Build history of the part. All positions in model axes, mm. Round coordinates to 2 decimals unless told otherwise and drop trailing zeros. Order: outer loops, then holes, each group sorted by start corner. A loop starts at its lowest first (then second) coordinate and runs counter-clockwise, first axis right, second up. Notation, with made-up numbers: (10.25, 9) -> (22.25, 9) arc R11 cw to (22.25, 17) -> close; hole circle Ø2 at (36.25, 58). An arc over 180 degrees is marked (long way). Use a Markdown table: item, result. Add a question column.
Item 1: Slice it at B-B, the plane x = 44.5. Give the cut face in (y, z).
Item 2: Slice it at A-A, the plane x = -4.5. Give the cut face in (y, z).
Item 3: Slice it at C-C, the plane y = -9.5. Give the cut face in (x, z), plus the area to 3 significant figures.
Item 4: Probe L1, parallel to Y at x = 60, z = 0.1; L2, parallel to X at y = -14, z = 0.55; L3, parallel to X at y = -26, z = 0.7. List the from-to ranges inside material, lowest first.
Item 5: Two-plate mould, pull along X, no slides. Class faces 1 (the face through (15.343, -16.242, 0.493)), 2 (the face through (-19.63, 22.23, 0.49)), 3 (the face through (12, -5, 1)): released by +X, released by -X, zero draft, split by the parting line, or undercut.
Item 6: Slice it at D-D, the plane z = 0.65. State how many separate pieces and enclosed holes the cut face has, plus the area to 3 significant figures.
from build123d import *

# Parameters (mm, degrees)
F0_R     = 3.25
F0_W     = 21
F0_H     = 10.2114447155
F0_W_2   = 19.5
F0_H_2   = 5.9798656802
F0_W_3   = 45
F1_DEPTH = 1


# Not quite as in the source:
# - a feature names something its author has since deleted; it is built from what else it names


with BuildPart() as f1:
    # F0 (on Top) → F1 (new body)
    with BuildSketch(Plane.XY):
        Polygon((85.2658590674, -26.4641552444), (85.2658590674, 13.2858447556), (68.2658590674, 13.2858447556), (68.2658590674, -1.2141552444), (68.2658590674, -11.42559996), (68.2658590674, -26.4641552444), (23.2658590674, -26.4641552444), (9.2658590674, -26.4641552444), (9.2658590674, -22.7141552444), (-10.2341409326, -22.7141552444), (-10.2341409326, -26.4641552444), (-24.2341409326, -26.4641552444), (-45.2341409326, -26.4641552444), (-45.2341409326, -11.42559996), (-45.2341409326, -1.2141552444), (-45.2341409326, 13.2858447556), (-59.2341409326, 13.2858447556), (-59.2341409326, -26.4641552444), (-59.2341409326, -36.4641552444), (-24.2341409326, -36.4641552444), (85.2658590674, -36.4641552444), align=None)
        with Locations((-52.2341409326, -19.4641552444)):
            Circle(F0_R, mode=Mode.SUBTRACT)
        with Locations((76.7658590674, -19.4641552444)):
            Circle(F0_R, mode=Mode.SUBTRACT)
        with Locations((-52.2341409326, -0.9641552444)):
            Circle(F0_R, mode=Mode.SUBTRACT)
        with Locations((76.7658590674, -0.9641552444)):
            Circle(F0_R, mode=Mode.SUBTRACT)
        with Locations((-34.7341409326, -6.3198776022)):
            Rectangle(F0_W, F0_H)
        with Locations((-0.4841409326, 5.2757775957)):
            Rectangle(F0_W_2, F0_H_2)
        with Locations((45.7658590674, -6.3198776022)):
            Rectangle(F0_W_3, F0_H)
        Polygon((-24.2341409326, 13.2858447556), (-10.2341409326, 13.2858447556), (-10.2341409326, 26.5358447556), (-59.2341409326, 26.5358447556), (-59.2341409326, 13.2858447556), (-45.2341409326, 13.2858447556), align=None)
        with Locations((-17.2341409326, 20.0358447556)):
            Circle(F0_R, mode=Mode.SUBTRACT)
        Polygon((85.2658590674, 13.2858447556), (85.2658590674, 26.2858447556), (9.2658590674, 26.2858447556), (9.2658590674, 13.2858447556), (23.2658590674, 13.2858447556), (68.2658590674, 13.2858447556), align=None)
        with Locations((15.7658590674, 20.7858447556)):
            Circle(F0_R, mode=Mode.SUBTRACT)
        with Locations((76.7658590674, 20.0358447556)):
            Circle(F0_R, mode=Mode.SUBTRACT)
        Polygon((-10.2341409326, 2.2858447556), (-10.2341409326, 8.2657104358), (-10.2341409326, 13.2858447556), (-24.2341409326, 13.2858447556), (-24.2341409326, -1.2141552444), (-24.2341409326, -11.42559996), (-24.2341409326, -26.4641552444), (-10.2341409326, -26.4641552444), (-10.2341409326, -22.7141552444), align=None)
        with Locations((-17.2341409326, -19.4641552444)):
            Circle(F0_R, mode=Mode.SUBTRACT)
        Polygon((23.2658590674, 13.2858447556), (9.2658590674, 13.2858447556), (9.2658590674, 8.2657104358), (9.2658590674, 2.2858447556), (9.2658590674, -22.7141552444), (9.2658590674, -26.4641552444), (23.2658590674, -26.4641552444), (23.2658590674, -11.42559996), (23.2658590674, -1.2141552444), align=None)
        with Locations((15.7658590674, -19.4641552444)):
            Circle(F0_R, mode=Mode.SUBTRACT)
    extrude(amount=F1_DEPTH)


solid = f1.part
Check sheet entries:
| question | item | result |
|---|---|---|
| 1 | outline | (-36.46, 0) -> (-26.46, 0) -> (-26.46, 1) -> (-36.46, 1) -> close; (-11.43, 0) -> (-1.21, 0) -> (-1.21, 1) -> (-11.43, 1) -> close; (13.29, 0) -> (26.29, 0) -> (26.29, 1) -> (13.29, 1) -> close |
| 2 | outline | (-36.46, 0) -> (-22.71, 0) -> (-22.71, 1) -> (-36.46, 1) -> close; (2.29, 0) -> (8.27, 0) -> (8.27, 1) -> (2.29, 1) -> close |
| 3 | outline | (-59.23, 0) -> (-10.23, 0) -> (-10.23, 1) -> (-59.23, 1) -> close; (9.27, 0) -> (85.27, 0) -> (85.27, 1) -> (9.27, 1) -> close |
| 3 | area | 125 mm2 |
| 4 | L1 | -36.46 to -26.46, -11.43 to -1.21, 13.29 to 26.29 |
| 4 | L2 | -59.23 to -45.23, -24.23 to -10.23, 9.27 to 23.27, 68.27 to 85.27 |
| 4 | L3 | -59.23 to -45.23, -24.23 to 23.27, 68.27 to 85.27 |
| 5 | face 1 | undercut |
| 5 | face 2 | undercut |
| 5 | face 3 | zero draft |
| 6 | separate pieces | 1 |
| 6 | enclosed holes | 14 |
| 6 | area | 5,990 mm2 |
